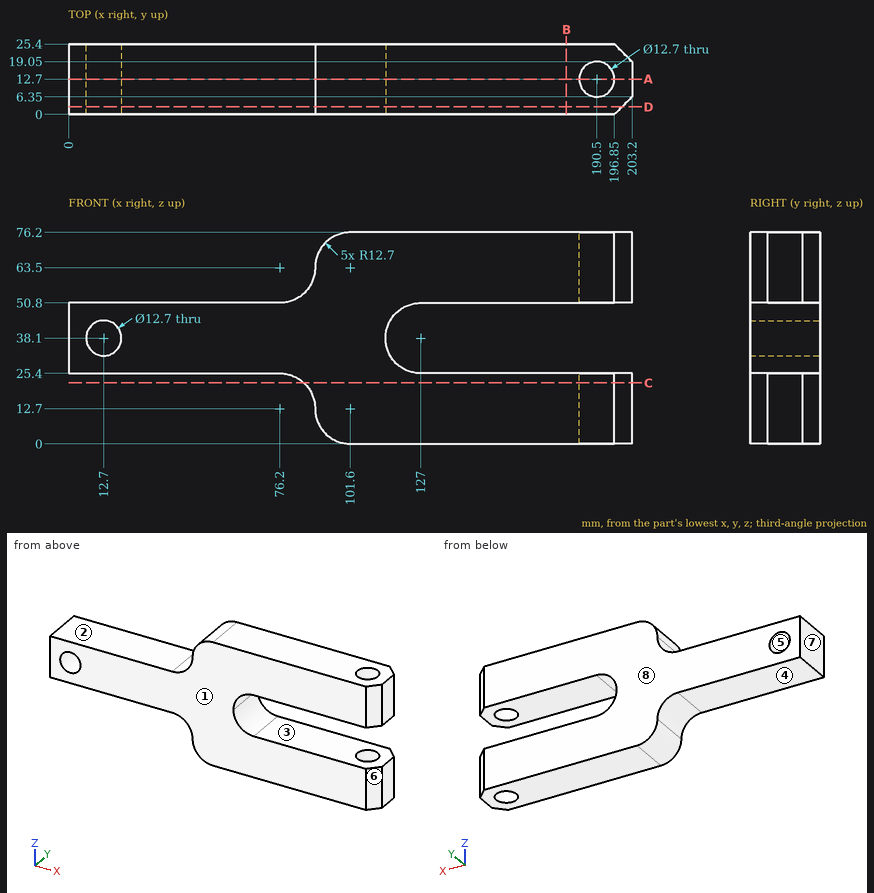
The drawing under review shows one solid part. Ordinate dimensions are in mm from its lowest x, y, z. A direction names the side the tool comes from. Give positions to 0.01 mm unless a question says otherwise; leave off trailing zeros. Order: outer loops, then holes, each group sorted by start corner. A loop starts at its lowest first (then second) coordinate and runs counter-clockwise, first axis right, second up. Notation, with made-up numbers: (-22.75, -5) - (6.25, -5) arc R25 cw to (6.25, 17) - close; hole circle Ø5 at (44, -26.5). An arc over 180 degrees is marked (long way). Answer as a JSON object with one key per item and string values. Group by question number.
Item 1: Clearance check with flat-ended pins moving along their axes: pin 1 Ø4 at (y, z) = (5, 10.5) entering from -X; pin 2 Ø5 at (x, y) = (44.5, 3.5) entering from -Z; pin 3 Ø5 at (y, z) = (5.5, 31.5) entering from +X. State where each tip first meets the part, or that it passes through.
Item 2: Draft analysis for pull direction X (two halves, no side actions). For the marked faces 5, 6, 7 and 8, state which applies: pulls with the +X half, pulls with the -X half, needs draft (parallel to the pull), parting line crosses it, or undercut.
Item 3: Take a section at A-A on y = 12.7. Give the boundary of the cut face in (x, z).
Item 4: Take a section at B-B on x = 179.5. Give the boundary of the cut face in (y, z).
Item 5: Take a section at C-C on z = 22. Give the boundary of the cut face in (x, y).
Item 6: Machinability: for the marked faces 1, 2, 3 and 4, which of the approach directions +Z, -Z, +X, -X, +Y, -Y give a long, thin tool a straight path to every point of the face, cutting with its end or side? Answer none if there is none.
Item 7: Take a section at D-D on y = 2.75. Give the boundary of the cut face in (x, z), and give its area (3 significant figures).
Item 8: Wall thickness on line 1 along Z through (x, y) = (12.7, 13); line 2 along Z through (x, y) = (190.5, 21.5); line 3 along Y through (x, z) = (190.5, 15.5): over which ranges is each line inside the solid? List them lowest first.
Reported:
{
 "1": {"pin 1": "x = 88.9", "pin 2": "z = 25.4", "pin 3": "x = 118.14"},
 "2": {"face 5": "undercut", "face 6": "pulls with the +X half", "face 7": "pulls with the -X half", "face 8": "needs draft"},
 "3": {"outline": "(0, 25.4) - (76.2, 25.4) arc R12.7 cw to (88.9, 12.7) arc R12.7 ccw to (101.6, 0) - (184.15, 0) - (184.15, 25.4) - (127, 25.4) arc R12.7 cw to (127, 50.8) - (184.15, 50.8) - (184.15, 76.2) - (101.6, 76.2) arc R12.7 ccw to (88.9, 63.5) arc R12.7 cw to (76.2, 50.8) - (0, 50.8) - close; (196.85, 0) - (203.2, 0) - (203.2, 25.4) - (196.85, 25.4) - close; (196.85, 50.8) - (203.2, 50.8) - (203.2, 76.2) - (196.85, 76.2) - close; hole circle Ø12.7 at (12.7, 38.1)"},
 "4": {"outline": "(0, 0) - (25.4, 0) - (25.4, 25.4) - (0, 25.4) - close; (0, 50.8) - (25.4, 50.8) - (25.4, 76.2) - (0, 76.2) - close"},
 "5": {"outline": "(84.85, 0) - (196.85, 0) - (203.2, 6.35) - (203.2, 19.05) - (196.85, 25.4) - (84.85, 25.4) - close; hole circle Ø12.7 at (190.5, 12.7)"},
 "6": {"face 1": "+Z, -Z, +X, -X, -Y", "face 2": "+Z, -X, +Y, -Y", "face 3": "+X, +Y, -Y", "face 4": "-Z, -X, +Y, -Y"},
 "7": {"outline": "(0, 25.4) - (76.2, 25.4) arc R12.7 cw to (88.9, 12.7) arc R12.7 ccw to (101.6, 0) - (199.6, 0) - (199.6, 25.4) - (127, 25.4) arc R12.7 cw to (127, 50.8) - (199.6, 50.8) - (199.6, 76.2) - (101.6, 76.2) arc R12.7 ccw to (88.9, 63.5) arc R12.7 cw to (76.2, 50.8) - (0, 50.8) - close; hole circle Ø12.7 at (12.7, 38.1)", "area": "8,470 mm^2"},
 "8": {"line 1": "25.4 to 31.75, 44.45 to 50.8", "line 2": "0 to 25.4, 50.8 to 76.2", "line 3": "0 to 6.35, 19.05 to 25.4"}
}
